from build123d import *

# Parameters (mm, degrees)
F2_SIZE = 1


with BuildPart() as f1:
    # F0 (on Front) → F1 (revolve)
    with BuildSketch(Plane.XZ):
        Polygon((-72.3989970755, 34.4926873816), (-72.3989970755, 19.4926873816), (-42.3989970755, 19.4926873816), (-42.3989970755, 17.4926873816), (-37.3989970755, 17.4926873816), (-37.3989970755, 30.4926873816), (-37.3989970755, 30.9926873816), (-35.3989970755, 30.9926873816), (-35.3989970755, 30.4926873816), (-27.3989970755, 30.4926873816), (-27.3989970755, 34.4926873816), align=None)
    revolve(axis=Axis((-49.8989970755, 0, 34.4926873816), (-1, 0, 0)))

    # F2
    f2_edges = [f1.edges().sort_by_distance(p)[0] for p in [
        (-37.398997, 0, 51.492687),
        (-42.398997, 0, 51.492687),
        (-72.398997, 0, 49.492687),
    ]]
    chamfer(f2_edges, length=F2_SIZE)


solid = f1.part
For this review, take the finished solid that the model builds, in its own axes (mm). A direction names the side the tool comes from. Give positions to 0.01 mm unless a question says otherwise; leave off trailing zeros. Order: outer loops, then holes, each group sorted by start corner. A loop starts at its lowest first (then second) coordinate and runs counter-clockwise, first axis right, second up. Notation, with made-up numbers: (-3.5, 67.5) - (50.5, 67.5) arc R4 ccw to (50.5, 73.5) - close; hole circle Ø4 at (24.25, 7). An arc over 180 degrees is marked (long way). Answer as a JSON object with one key per item and string values. Group by question number.
Item 1: Clearance check with flat-ended pins moving along their axes: pin 1 Ø2 at (x, y) = (-59, -6.5) entering from +Z; pin 2 Ø1 at (x, z) = (-43.5, 25.5) entering from +Y; pin 3 Ø1.5 at (x, y) = (-64, 12) entering from -Z. State where each tip first meets the part, or that it passes through.
Item 2: Take a section at C-C on x = -36. Give the boundary of the cut face in (y, z), and give its area (3 significant figures).
Item 3: Take a section at B-B on x = -54.5. Give the boundary of the cut face in (y, z).
Item 4: Take a section at A-A on y = 0. Give the boundary of the cut face in (x, z).
Item 5: Wall thickness on line 1 along X through (y, z) = (-2, 31.5); line 2 along X through (y, z) = (13, 31.5); line 3 along X through (y, z) = (-8, 47.5): over which ranges is each line inside the solid? List them lowest first.
Item 6: Machinability: for faces 1 (the cylindrical face through (-39.878, -0.747, 51.476)), 2 (the cylindrical face through (-56.696, 14.643, 37.744)), which of the approach directions +Z, -Z, +X, -X, +Y, -Y give a long, thin tool a straight path to every point of the face, cutting with its end or side? Answer none if there is none.
Item 7: Draft analysis for pull direction X (two halves, no side actions). For faces 3 (the flat face through (-72.399, 0, 34)), 4 (the cylindrical face through (-31.343, -1.201, 30.677)), 5 (the flat face through (-27.399, 0, 35)), 6 (the cylindrical face through (-36.38, -0.15, 37.99)), state which applies: pulls with the +X half, pulls with the -X half, needs draft (parallel to the pull), parting line crosses it, or undercut.
Reported:
{
 "1": {"pin 1": "z = 48.45", "pin 2": "y = 12.36", "pin 3": "z = 24.57"},
 "2": {"outline": "circle Ø7 at (0, 34.49)", "area": "38.5 mm^2"},
 "3": {"outline": "circle Ø30 at (0, 34.49)"},
 "4": {"outline": "(-72.4, 20.49) - (-71.4, 19.49) - (-42.4, 19.49) - (-42.4, 18.49) - (-41.4, 17.49) - (-38.4, 17.49) - (-37.4, 18.49) - (-37.4, 30.99) - (-35.4, 30.99) - (-35.4, 30.49) - (-27.4, 30.49) - (-27.4, 38.49) - (-35.4, 38.49) - (-35.4, 37.99) - (-37.4, 37.99) - (-37.4, 50.49) - (-38.4, 51.49) - (-41.4, 51.49) - (-42.4, 50.49) - (-42.4, 49.49) - (-71.4, 49.49) - (-72.4, 48.49) - close"},
 "5": {"line 1": "-72.4 to -37.4, -35.4 to -27.4", "line 2": "-72.4 to -37.4", "line 3": "-42.4 to -37.4"},
 "6": {"face 1": "+X, -X", "face 2": "-X"},
 "7": {"face 3": "pulls with the -X half", "face 4": "needs draft", "face 5": "pulls with the +X half", "face 6": "undercut"}
}
